from build123d import *

# Parameters (mm, degrees)
SKETCH_1_W          = 20
SKETCH_1_H          = 18
EXTRUDE_1_DEPTH     = 3
SKETCH_2_W          = 4
SKETCH_2_H          = 18
EXTRUDE_2_DEPTH     = 12
SKETCH_4_R          = 1
CUT_EXTRUDE_1_DEPTH = 35.263683398
SKETCH_5_R          = 1
CUT_EXTRUDE_2_DEPTH = 5
SKETCH_6_W          = 4
SKETCH_6_H          = 12
EXTRUDE_3_DEPTH     = 25
SKETCH_7_W          = 4
SKETCH_7_H          = 12
EXTRUDE_4_DEPTH     = 25
SKETCH_8_R          = 1.2
CUT_EXTRUDE_3_DEPTH = 4


with BuildPart() as part:
    # 草图1 → 凸台-拉伸1 (new body)
    with BuildSketch(Plane(origin=(0, 0, 0), x_dir=(1, 0, 0), z_dir=(0, 1, 0))):
        with Locations((15, -9)):
            Rectangle(SKETCH_1_W, SKETCH_1_H)
    extrude(amount=EXTRUDE_1_DEPTH)

    # 草图2 → 凸台-拉伸2 (add)
    with BuildSketch(Plane(origin=(0, 3, 0), x_dir=(1, 0, 0), z_dir=(0, 1, 0))):
        with Locations((23, -9)):
            Rectangle(SKETCH_2_W, SKETCH_2_H)
    extrude(amount=EXTRUDE_2_DEPTH)

    # 草图4 → 切除-拉伸1 (cut, through all)
    with BuildSketch(Plane.XZ):
        with Locations(Location((17.75, 15, 0), (0, 0, 270))):
            Circle(SKETCH_4_R)
        with Locations(Location((17.75, 3, 0), (0, 0, 270))):
            Circle(SKETCH_4_R)
        with Locations(Location((9.75, 3, 0), (0, 0, 270))):
            Circle(SKETCH_4_R)
        with Locations(Location((9.75, 15, 0), (0, 0, 270))):
            Circle(SKETCH_4_R)
    extrude(amount=-CUT_EXTRUDE_1_DEPTH, mode=Mode.SUBTRACT)

    # 草图5 → 切除-拉伸2 (cut)
    with BuildSketch(Plane(origin=(0, 15, 0), x_dir=(1, 0, 0), z_dir=(0, 1, 0))):
        with Locations(Location((23, -15, 0), (0, 0, 270))):
            Circle(SKETCH_5_R)
        with Locations(Location((23, -3, 0), (0, 0, 270))):
            Circle(SKETCH_5_R)
    extrude(amount=-CUT_EXTRUDE_2_DEPTH, mode=Mode.SUBTRACT)

    # 草图6 → 凸台-拉伸3 (add)
    with BuildSketch(Plane.XY.offset(18)):
        with Locations((23, 9)):
            Rectangle(SKETCH_6_W, SKETCH_6_H)
    extrude(amount=EXTRUDE_3_DEPTH)

    # 草图7 → 凸台-拉伸4 (add)
    with BuildSketch(Plane(origin=(0, 0, 0), x_dir=(-1, 0, 0), z_dir=(0, 0, -1))):
        with Locations((-23, 9)):
            Rectangle(SKETCH_7_W, SKETCH_7_H)
    extrude(amount=EXTRUDE_4_DEPTH)

    # 草图8 → 切除-拉伸3 (cut)
    with BuildSketch(Plane.ZY.offset(-21)):
        with Locations((-36, 11.5)):
            Circle(SKETCH_8_R)
        with Locations((-21, 11.5)):
            Circle(SKETCH_8_R)
        with Locations((9, 11.5)):
            Circle(SKETCH_8_R)
        with Locations((24, 11.5)):
            Circle(SKETCH_8_R)
    extrude(amount=-CUT_EXTRUDE_3_DEPTH, mode=Mode.SUBTRACT)


solid = part.part
The listing builds one solid part. Answer for the finished solid, in the listing's coordinates (mm). A direction names the side the tool comes from. Give positions to 0.01 mm unless a question says otherwise; leave off trailing zeros. Loops run counter-clockwise (first coordinate to the right, second up) from the corner with the lowest first, then second, coordinate; pieces in that order, holes last.
Item 1: A cutting plane is placed at A-A (z = 24). Give the vertices of the cut face in (x, y), then the cut area to 3 significant figures.
Derived:
outline: (21, 3) - (25, 3) - (25, 10.3) - (21, 10.3) - close; (21, 12.7) - (25, 12.7) - (25, 15) - (21, 15) - close
area: 38.4 mm2
Item 2: A cutting plane is placed at B-B (y = 11.5). Give the vertices of the cut face in (x, z).
Derived:
outline: (21, -25) - (25, -25) - (25, -22.2) - (21, -22.2) - close; (21, -19.8) - (25, -19.8) - (25, 7.8) - (21, 7.8) - close; (21, 10.2) - (25, 10.2) - (25, 22.8) - (21, 22.8) - close; (21, 25.2) - (25, 25.2) - (25, 43) - (21, 43) - close; hole circle Ø2 at (23, 3); hole circle Ø2 at (23, 15)
Item 3: Find the intervals of material crossed by line 1 along X through (y, z) = (1.65, 15); line 2 along Y through (x, z) = (22.75, -21); line 3 along X through (y, z) = (11.25, 15), in increasing order.
Derived:
line 1: x = 5 to 8.75, 10.75 to 16.75, 18.75 to 25
line 2: y = 3 to 10.3, 12.7 to 15
line 3: x = 21 to 22, 24 to 25
Item 4: Determine the mould class of faces 5 (the flat face through (13, 3, 9)), 6 (the flat face through (15, 1, 18)), 7 (the flat face through (23, 10, 3)) for opening direction Z: +Z half, -Z half, draft (parallel to the pull), parting line (faces both ways), or undercut.
Derived:
face 5: draft
face 6: +Z half
face 7: undercut
Item 5: A cutting plane is placed at C-C (x = 9.75). Give the vertices of the cut face in (y, z).
Derived:
outline: (0, 0) - (3, 0) - (3, 2) - (0, 2) - close; (0, 4) - (3, 4) - (3, 14) - (0, 14) - close; (0, 16) - (3, 16) - (3, 18) - (0, 18) - close
Item 6: Each of these flat-tipped pins is pushed along its axis until it touches: pin 1 Ø3 at (x, z) = (9.75, 15) entering from +Y; pin 2 Ø1.8 at (x, z) = (17.75, 15) entering from -Y; pin 3 Ø4.5 at (x, z) = (22.5, -9.5) entering from -Y; pin 4 Ø4 at (y, z) = (3.5, 33) entering from -X. Where does it stop, or does it pass through?
Derived:
pin 1: stops at y = 3
pin 2: passes through
pin 3: stops at y = 3
pin 4: stops at x = 21
Item 7: A tool of negligible diameter and unlimited length cuts with its end or side. For faces 1 (the cylindrical face through (22, 13, 3)), 2 (the flat face through (23, 3, -12)), 3 (the flat face through (23, 3, 30)), 4 (the flat face through (21, 9, 9)), from which of +Z, -Z, +X, -X, +Y, -Y can it reach the whole face along a straight path? Write none if from no direction.
Derived:
face 1: +Y
face 2: -Z, +X, -X, -Y
face 3: +Z, +X, -X, -Y
face 4: +Z, -Z, -X, +Y
Item 8: A cutting plane is placed at D-D (x = 23). Give the vertices of the cut face in (y, z), then the cut area to 3 significant figures.
Derived:
outline: (0, 0) - (3, 0) - (3, -25) - (15, -25) - (15, 2) - (10, 2) - (10, 4) - (15, 4) - (15, 14) - (10, 14) - (10, 16) - (15, 16) - (15, 43) - (3, 43) - (3, 18) - (0, 18) - close; hole circle Ø2.4 at (11.5, -21); hole circle Ø2.4 at (11.5, 9); hole circle Ø2.4 at (11.5, 24)
area: 836 mm2
